Autodesk Inventor part; units mm, degrees
ref_plane "YZ Plane" through (0, 0, 0) normal (1, 0, 0) x (0, 1, 0)
ref_plane "XZ Plane" through (0, 0, 0) normal (0, 1, 0) x (-1, 0, 0)
ref_plane "XY Plane" through (0, 0, 0) normal (0, 0, 1) x (1, 0, 0)
sketch "Boceto2" plane through (0, 0, 0) normal (0, 1, 0) x (-1, 0, 0)
  line L0 (33.18, 42.36) -> (-33.18, 42.36)
  line L1 (-33.18, 42.36) -> (-33.18, -42.36)
  line L2 (-33.18, -42.36) -> (33.18, -42.36)
  line L3 (33.18, -42.36) -> (33.18, 42.36)
  line L4 (33.18, 42.36) -> (-33.18, -42.36) construction
  line L5 (-33.18, 42.36) -> (33.18, -42.36) construction
  line L6 (15, 42.36) -> (-15, 42.36)
  line L7 (-15, 42.36) -> (-15, 39.18)
  line L8 (-15, 39.18) -> (15, 39.18)
  line L9 (15, 39.18) -> (15, 42.36)
  line L10 (15, 42.36) -> (-15, 39.18) construction
  line L11 (-15, 42.36) -> (15, 39.18) construction
  line L12 (15, 9.18) -> (-15, 9.18)
  line L13 (-15, 9.18) -> (-15, 6)
  line L14 (-15, 6) -> (15, 6)
  line L15 (15, 6) -> (15, 9.18)
  line L16 (15, 9.18) -> (-15, 6) construction
  line L17 (-15, 9.18) -> (15, 6) construction
  line L18 (15, -24) -> (-15, -24)
  line L19 (-15, -24) -> (-15, -27.18)
  line L20 (-15, -27.18) -> (15, -27.18)
  line L21 (15, -27.18) -> (15, -24)
  line L22 (15, -24) -> (-15, -27.18) construction
  line L23 (-15, -24) -> (15, -27.18) construction
  line L24 (15, -39.18) -> (-15, -39.18)
  line L25 (-15, -39.18) -> (-15, -42.36)
  line L26 (-15, -42.36) -> (15, -42.36)
  line L27 (15, -42.36) -> (15, -39.18)
  line L28 (15, -39.18) -> (-15, -42.36) construction
  line L29 (-15, -39.18) -> (15, -42.36) construction
  line L30 (-30, 25) -> (-33.18, 25)
  line L31 (-33.18, 25) -> (-33.18, -25)
  line L32 (-33.18, -25) -> (-30, -25)
  line L33 (-30, -25) -> (-30, 25)
  line L34 (-30, 25) -> (-33.18, -25) construction
  line L35 (-33.18, 25) -> (-30, -25) construction
  line L36 (33.18, 25) -> (30, 25)
  line L37 (30, 25) -> (30, -25)
  line L38 (30, -25) -> (33.18, -25)
  line L39 (33.18, -25) -> (33.18, 25)
  line L40 (33.18, 25) -> (30, -25) construction
  line L41 (30, 25) -> (33.18, -25) construction
  line L42 (30, 3.5) -> (0, 3.5)
  line L43 (0, 3.5) -> (0, -21.5)
  line L44 (0, -21.5) -> (30, -21.5)
  line L45 (30, -21.5) -> (30, 3.5)
  line L46 (30, 3.5) -> (0, -21.5) construction
  line L47 (0, 3.5) -> (30, -21.5) construction
  point P0 (0, 0)
  point P1 (0, 40.77)
  point P2 (0, 7.59)
  point P3 (0, -25.59)
  point P4 (0, -40.77)
  point P5 (-31.59, 0)
  point P6 (31.59, 0)
  point P7 (15, -9)
  dimension "d37" = 84.72
  dimension "d38" = 66.36
  dimension "d39" = 30
  dimension "d40" = 3.18
  dimension "d41" = 0
  dimension "d42" = 3.18
  dimension "d43" = 30
  dimension "d44" = 30
  dimension "d45" = 3.18
  dimension "d46" = 30
  dimension "d47" = 30
  dimension "d48" = 12
  dimension "d49" = 50
  dimension "d50" = 0
  dimension "d51" = 0
  dimension "d52" = 50
  dimension "d53" = 15
  dimension "d54" = 25
  dimension "d59" = 30
extrude "Extrusión2" add sketch "Boceto2" along normal blind 3.18 contours L3 L36 L37 L42 L43 L44 L38 L2 L27 L24 L25 L1 L32 L33 L30 L0 L7 L8 L9
properties part number "HOMBRO_TAPA.LAT"
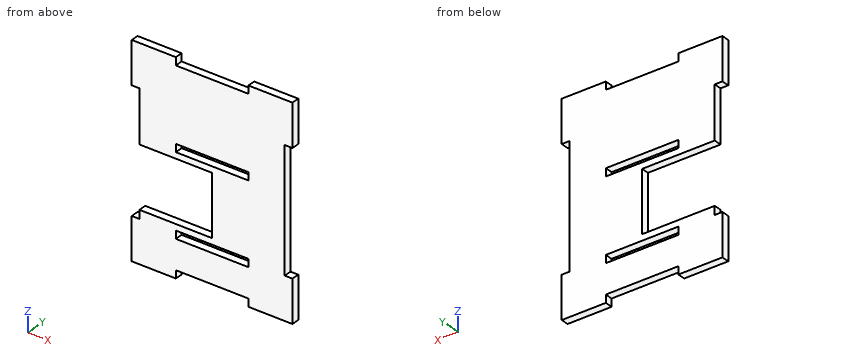
Check sheet for the modelled part. Datum: model origin and axes. Units: mm. Give positions to 0.01 mm unless a question says otherwise; leave off trailing zeros. Order: outer loops, then holes, each group sorted by start corner. A loop starts at its lowest first (then second) coordinate and runs counter-clockwise, first axis right, second up. Notation, with made-up numbers: (-24.75, 83.25) -> (15.25, 83.25) arc R24 cw to (15.25, 96.25) -> close; hole circle Ø7 at (30, 10.5). An arc over 180 degrees is marked (long way). Return JSON: item names as keys, results as strings.
1. Cross-section at C-C, the plane y = 1.3. Count the separate pieces of the cut face and the enclosed holes in it, plus the area to 3 significant figures.
From the geometry:
{"separate pieces": "1", "enclosed holes": "2", "area": "4,170 mm^2"}
2. Cross-section at A-A, the plane x = 4. Record the cut outline in (y, z).
From the geometry:
{"outline": "(0, -39.18) -> (3.18, -39.18) -> (3.18, -27.18) -> (0, -27.18) -> close; (0, -24) -> (3.18, -24) -> (3.18, 6) -> (0, 6) -> close; (0, 9.18) -> (3.18, 9.18) -> (3.18, 39.18) -> (0, 39.18) -> close"}
3. Go/stop test with flat-tipped pins: P1, Ø1.6, axis at x = 6.5, y = 1, coming from the +Z side; P2, Ø1.6, axis at y = 1, z = -8.5, coming from the -X side. Record where each tip stops, or that it passes through.
From the geometry:
{"P1": "z = 39.18", "P2": "x = 0"}
4. Material ranges on probe 1 along Z at (x, y) = (-9, 0.6); probe 2 along Z at (x, y) = (14, 0.1); probe 3 along X at (y, z) = (2.2, 7.5), recorded low to high. Write a range as [from, to].
From the geometry:
{"probe 1": "[-39.18, -27.18], [-24, -21.5], [3.5, 6], [9.18, 39.18]", "probe 2": "[-39.18, -27.18], [-24, 6], [9.18, 39.18]", "probe 3": "[-30, -15], [15, 30]"}
5. Cross-section at B-B, the plane x = -3.5. Record the cut outline in (y, z), plus the area to 3 significant figures.
From the geometry:
{"outline": "(0, -39.18) -> (3.18, -39.18) -> (3.18, -27.18) -> (0, -27.18) -> close; (0, -24) -> (3.18, -24) -> (3.18, -21.5) -> (0, -21.5) -> close; (0, 3.5) -> (3.18, 3.5) -> (3.18, 6) -> (0, 6) -> close; (0, 9.18) -> (3.18, 9.18) -> (3.18, 39.18) -> (0, 39.18) -> close", "area": "149 mm^2"}
6. Cross-section at D-D, the plane x = -26. Record the cut outline in (y, z), plus the area to 3 significant figures.
From the geometry:
{"outline": "(0, -42.36) -> (3.18, -42.36) -> (3.18, -21.5) -> (0, -21.5) -> close; (0, 3.5) -> (3.18, 3.5) -> (3.18, 42.36) -> (0, 42.36) -> close", "area": "190 mm^2"}
